The figure shows three views and two pictorial views of one solid part (mm, origin at its lowest corner). Answer the questions. Coordinates: 2 decimals unless noted, no trailing zeros. Loops run counter-clockwise (first coordinate to the right, second up) from the corner with the lowest first, then second, coordinate; pieces in that order, holes last. Notation, with made-up numbers: M 42.5,74.5 L 91.5,74.5 A25 ccw 91.5,100.5 Z; hole C -30.75,8 d3. An arc over 180 degrees is marked long. Return JSON: item names as keys, results as strings. Group by question number.
1. Section B-B (y = 1.5) is taken. Write down the section's boundary in (x, z), then the cut area to 3 significant figures.
2. Section C-C (z = 3.5) is taken. Write down the section's boundary in (x, y).
3. Straight lines are drawn through the part: L1, parallel to X at y = 5.75, z = 9.25; L2, parallel to X at y = 0.5, z = 9; L3, parallel to Z at x = 44, y = 2. For each, find the intervals that lie inside material, in ascending order. Write a range as from..to.
4. Section A-A (x = 24) is taken. Write down the section's boundary in (y, z).
5. Section D-D (x = 35.5) is taken. Write down the section's boundary in (y, z).
6. The mould has two halves that part along X. Classify the marked faces 1, 2 and 3: pulls with the +X half, pulls with the -X half, needs draft (parallel to the pull), parting line crosses it, or undercut.
7. Given P1, Ø0.8, axis at x = 7.5, y = 7.5, coming from the +Z side; P2, Ø2, axis at y = 7, z = 8, coming from the -X side; P3, Ø1.5, axis at x = 50, y = 1, coming from the -Z side; P4, Ø2.5, axis at x = 42, z = 3, coming from the -Y side, each flat-ended and moving along its own axis, determine where each tip first touches the part or whether it passes through.
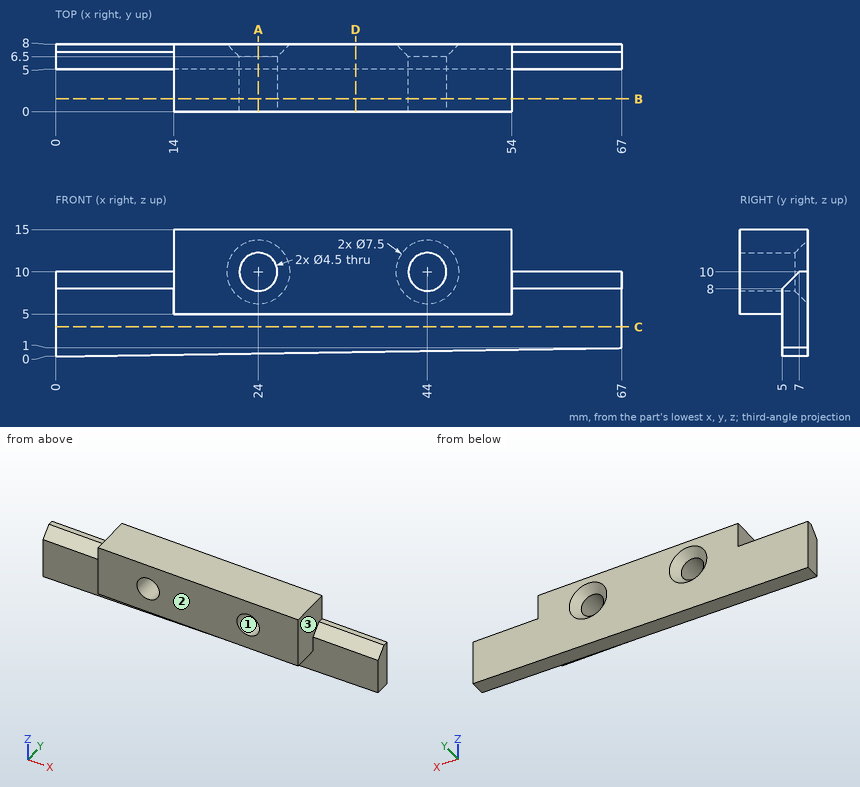
Worked out:
{
 "1": {"outline": "M 14,5 L 54,5 L 54,15 L 14,15 Z; hole C 24,10 d4.5; hole C 44,10 d4.5", "area": "368 mm^2"},
 "2": {"outline": "M 0,5 L 67,5 L 67,8 L 0,8 Z"},
 "3": {"L1": "14..21.88, 26.12..41.88, 46.12..54", "L2": "14..21.98, 26.02..41.98, 46.02..54", "L3": "5..7.75, 12.25..15"},
 "4": {"outline": "M 0,5 L 5,5 L 5,0.36 L 8,0.36 L 8,6.25 L 6.5,7.75 L 0,7.75 Z; M 0,12.25 L 6.5,12.25 L 8,13.75 L 8,15 L 0,15 Z"},
 "5": {"outline": "M 0,5 L 5,5 L 5,0.53 L 8,0.53 L 8,15 L 0,15 Z"},
 "6": {"face 1": "undercut", "face 2": "needs draft", "face 3": "pulls with the +X half"},
 "7": {"P1": "z = 10", "P2": "x = 0", "P3": "z = 5", "P4": "y = 5"}
}
